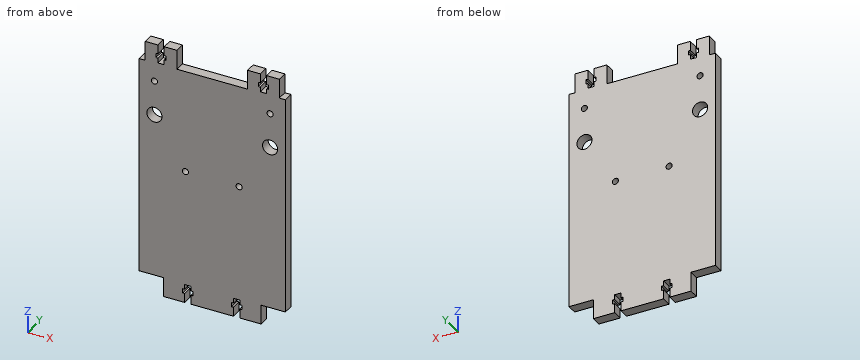
```python
from build123d import *

# Parameters (mm, degrees)
F0_W      = 76.2
F0_H      = 134.62
F1_DEPTH  = 5.334
F2_W      = 12.7
F2_H      = 10.16
F3_DEPTH  = 25.4
F4_W      = 3.302
F4_H      = 4.826
F4_H_2    = 2.286
F4_W_2    = 1.0414
F4_H_3    = 2.54
F5_DEPTH  = 25.4
F6_W      = 3.175
F6_H      = 10.16
F6_W_2    = 36.83
F7_DEPTH  = 25.4
F8_W      = 3.302
F8_H      = 4.826
F8_H_2    = 2.286
F8_H_3    = 2.54
F8_W_2    = 1.0414
F9_DEPTH  = 25.4
F10_R     = 1.6
F10_R_2   = 3.935
F11_DEPTH = 25.4


with BuildPart() as f1:
    # F0 (on Front) → F1 (new body)
    with BuildSketch(Plane.XZ):
        with Locations((11.8567193806, 14.6954228854)):
            Rectangle(F0_W, F0_H)
    extrude(amount=F1_DEPTH)

    # F2 (on face) → F3 (cut)
    with BuildSketch(Plane.XZ.offset(5.334)):
        with Locations((-19.8932806194, -47.5345771146)):
            Rectangle(F2_W, F2_H)
        with Locations((43.6067193806, -47.5345771146)):
            Rectangle(F2_W, F2_H)
    extrude(amount=-F3_DEPTH, mode=Mode.SUBTRACT)

    # F4 (on face) → F5 (cut)
    with BuildSketch(Plane.XZ.offset(5.334)):
        with Locations((-0.8432806194, -50.2015771146)):
            Rectangle(F4_W, F4_H)
        with Locations((-0.8432806194, -46.6455771146)):
            Rectangle(F4_W, F4_H_2)
        with Locations((-3.0149806194, -46.6455771146)):
            Rectangle(F4_W_2, F4_H_2)
        with Locations((-0.8432806194, -44.2325771146)):
            Rectangle(F4_W, F4_H_3)
        with Locations((1.3284193806, -46.6455771146)):
            Rectangle(F4_W_2, F4_H_2)
        with Locations((24.5567193806, -50.2015771146)):
            Rectangle(F4_W, F4_H)
        with Locations((24.5567193806, -46.6455771146)):
            Rectangle(F4_W, F4_H_2)
        with Locations((22.3850193806, -46.6455771146)):
            Rectangle(F4_W_2, F4_H_2)
        with Locations((26.7284193806, -46.6455771146)):
            Rectangle(F4_W_2, F4_H_2)
        with Locations((24.5567193806, -44.2325771146)):
            Rectangle(F4_W, F4_H_3)
    extrude(amount=-F5_DEPTH, mode=Mode.SUBTRACT)

    # F6 (on face) → F7 (cut)
    with BuildSketch(Plane.XZ.offset(5.334)):
        with Locations((-24.6557806194, 76.9254228854)):
            Rectangle(F6_W, F6_H)
        with Locations((11.8567193806, 76.9254228854)):
            Rectangle(F6_W_2, F6_H)
        with Locations((48.3692193806, 76.9254228854)):
            Rectangle(F6_W, F6_H)
    extrude(amount=-F7_DEPTH, mode=Mode.SUBTRACT)

    # F8 (on face) → F9 (cut)
    with BuildSketch(Plane.XZ.offset(5.334)):
        with Locations((-14.8132806194, 79.5924228854)):
            Rectangle(F8_W, F8_H)
        with Locations((-14.8132806194, 76.0364228854)):
            Rectangle(F8_W, F8_H_2)
        with Locations((-14.8132806194, 73.6234228854)):
            Rectangle(F8_W, F8_H_3)
        with Locations((-16.9849806194, 76.0364228854)):
            Rectangle(F8_W_2, F8_H_2)
        with Locations((-12.6415806194, 76.0364228854)):
            Rectangle(F8_W_2, F8_H_2)
        with Locations((38.5267193806, 73.6234228854)):
            Rectangle(F8_W, F8_H_3)
        with Locations((38.5267193806, 76.0364228854)):
            Rectangle(F8_W, F8_H_2)
        with Locations((36.3550193806, 76.0364228854)):
            Rectangle(F8_W_2, F8_H_2)
        with Locations((40.6984193806, 76.0364228854)):
            Rectangle(F8_W_2, F8_H_2)
        with Locations((38.5267193806, 79.5924228854)):
            Rectangle(F8_W, F8_H)
    extrude(amount=-F9_DEPTH, mode=Mode.SUBTRACT)

    # F10 (on face) → F11 (cut)
    with BuildSketch(Plane.XZ.offset(5.334)):
        with Locations((-18.2432806194, 62.0054228854)):
            Circle(F10_R)
        with Locations((41.9567193806, 62.0054228854)):
            Circle(F10_R)
        with Locations((-18.2432806194, 43.9054228854)):
            Circle(F10_R_2)
        with Locations((41.9567193806, 43.9054228854)):
            Circle(F10_R_2)
        with Locations((-2.1132806194, 18.0054228854)):
            Circle(F10_R)
        with Locations((25.8267193806, 18.0054228854)):
            Circle(F10_R)
    extrude(amount=-F11_DEPTH, mode=Mode.SUBTRACT)


solid = f1.part
```
Part model, mm, in its own coordinate system. Round coordinates to 2 decimals unless told otherwise and drop trailing zeros. Order: outer loops, then holes, each group sorted by start corner. A loop starts at its lowest first (then second) coordinate and runs counter-clockwise, first axis right, second up. Notation, with made-up numbers: M 88.5,8 L 131.5,8 A24 ccw 131.5,47 Z; hole C -13.5,-6.5 d5. An arc over 180 degrees is marked long. Put each result on its own line as item: value. Start each with the question number.
1. Slice it at B-B on y = -2.15. State how many separate pieces and enclosed holes the cut face has, then the cut area to 3 significant figures.
2. Slice it at A-A on x = 19. List the corners of the cut face in (y, z), then the cut area to 3 significant figures.
3. Drop flat-ended pins along their axis: pin 1 (0.7 mm diameter, centred on y = -2.5, z = -46.5, fed in from -X); pin 2 (3 mm diameter, centred on y = -3, z = 73.5, fed in from -X); pin 3 (1.7 mm diameter, centred on x = 38.5, y = -4, fed in from +Z). Give the stop position or say it passes through.
4. Drill centre lines: probe 1 along X at (y, z) = (-5.1, 75); probe 2 along Z at (x, y) = (42, -0.4); probe 3 along Z at (x, y) = (-3.5, -2.65). Where is each one in solid material? Low to high. Write a range as [from, to].
Findings:
1. separate pieces: 1
1. enclosed holes: 6
1. area: 9,290 mm2
2. outline: M -5.33,-52.61 L 0,-52.61 L 0,71.85 L -5.33,71.85 Z
2. area: 664 mm2
3. pin 1: x = -13.54
3. pin 2: x = -23.07
3. pin 3: z = 72.35
4. probe 1: [-23.07, -17.51], [-12.12, -6.56], [30.27, 35.83], [41.22, 46.78]
4. probe 2: [-42.45, 39.97], [47.84, 60.41], [63.6, 82.01]
4. probe 3: [-52.61, -47.79], [-45.5, 17.21], [18.8, 71.85]
